Verification items for the finished model (mm, model axes). Face numbers are marked on the shaded views. A direction names the side the tool comes from. Round coordinates to 2 decimals unless told otherwise and drop trailing zeros. Loops run counter-clockwise (first coordinate to the right, second up) from the corner with the lowest first, then second, coordinate; pieces in that order, holes last. Notation, with made-up numbers: (29.5, 42) - (75.5, 42) arc R26 cw to (75.5, 74) - close; hole circle Ø6 at (61, 62.5). An arc over 180 degrees is marked (long way). Use CSV: the item, a comma, the result in double quotes.
Autodesk Inventor part; units mm, degrees
ref_plane "Work Plane1" through (1.525, 0, 0) normal (0, 0, 1) x (1, 0, 0)
ref_plane "YZ Plane" through (0, 0, 0) normal (1, 0, 0) x (0, 1, 0)
ref_plane "XZ Plane" through (0, 0, 0) normal (0, 1, 0) x (-1, 0, 0)
sketch "Sketch1" plane through (0, 0, 0) normal (0, 0, 1) x (1, 0, 0)
  line L0 (0, 14.1) -> (0, 10)
  line L1 (49, 10) -> (95, 10)
  line L2 (95, 10) -> (95, 0)
  line L3 (95, 0) -> (-0.8001, 0)
  line L4 (-19.9601, 0) -> (114.16, 0)
  line L5 (-0.8001, 0) -> (-0.8001, 14.1)
  line L6 (-0.8001, 14.1) -> (0, 14.1)
  line L7 (49, 10) -> (47.4663, 10)
  line L8 (47.4663, 10) -> (0, 10)
  line L9 (0, -2.82) -> (0, 16.92)
  dimension "d0" = 95
  dimension "d1" = 46
  dimension "d2" = 20
  dimension "d9" = 0.8001
  dimension "d10" = 28.2
  dimension "d13" = 1.5337
  dimension "d14" = 20
revolve "Body" add sketch "Sketch1" angle 360 about axis through (95, 0, 0) along (-1, 0, 0)
sketch "Sketch2" plane through (-0.8001, 0, 0) normal (-1, 0, 0) x (0, 0, 1)
  line L0 (0, 17.3205) -> (15, 8.6603)
  line L1 (15, 8.6603) -> (15, -8.6603)
  line L2 (15, -8.6603) -> (0, -17.3205)
  line L3 (0, -17.3205) -> (-15, -8.6603)
  line L4 (-15, -8.6603) -> (-15, 8.6603)
  line L5 (-15, 8.6603) -> (0, 17.3205)
  point P0 (0, 0)
  point P1 (0, 0)
  dimension "d11" = 30
extrude "Head" add sketch "Sketch2" along normal blind 11.7
sketch "Sketch4" plane through (0, 0, 0) normal (0, 0, 1) x (1, 0, 0)
  line L0 (-12.5001, 15) -> (-12.5001, 17.3205)
  line L1 (-12.5001, 17.3205) -> (-11.1604, 17.3205)
  line L2 (-11.1604, 17.3205) -> (-12.5001, 15)
  line L3 (-14.8401, 0) -> (1.5399, 0)
  line L4 (-0.8001, 17.3205) -> (-12.5001, 17.3205)
  line L5 (-12.5001, 8.6603) -> (-12.5001, 17.3205)
  dimension "d5" = 30
  dimension "d19" = 30
revolve "Chamfer1" cut sketch "Sketch4" angle 360 about axis through (-10, 0, 0) along (1, 0, 0)
thread "Thread"
chamfer "Chamfer2" distance 1.5336 distance2 1.5337 1 edges at (95, -10, 0) measured on face at (95, -2.495, 2.2104)
ref_plane "Work Plane1" through (1.525, 0, 0) normal (0, 0, 1) x (1, 0, 0)
equation "\"d0\" = NLG"
equation "\"d1\" = GEL"
equation "\"d2\" = GD"
equation "\"d10\" = SD2"
equation "\"d14\" = BDM"
equation "\"d11\" = SW"
equation "\"d3\" = KOH - SD"
equation "\"d5\" = ANG1"
equation "\"d19\" = SW0"
equation "\"d15\" = GEL"
equation "\"d6\" = -0.5 * SPD + 0.5 * GD"
equation "\"NLG\" = 95"
equation "\"GD\" = NND"
equation "\"BDM\" = NND"
equation "\"KOH\" = 12.5"
equation "\"GEL\" = 46"
equation "\"SW\" = 30"
equation "\"SW0\" = SW"
equation "\"SPD\" = NND - 1.2269 * PTC"
equation "\"SD2\" = 28.2"
equation "\"SD\" = 0.8"
equation "\"ANG1\" = 30deg"
equation "\"GAL\" = 0.61345 * PTC"
equation "\"GUL\" = 0.61345 * PTC"
equation "\"RR\" = 0.8"
equation "\"WFT\" = SD"
equation "\"GD1\" = THREADDIA - 1.2269 * PTC"
equation "\"SDH\" = 28.2"
equation "\"TOA\" = 30deg"
equation "\"FAWI\" = 45deg"
equation "\"PTC\" = 2.5"
equation "\"E0\" = 1.155 * SW"
properties part number "Bolt M20x95-8.8-A PN-85/M-82101" material "Steel, Mild"
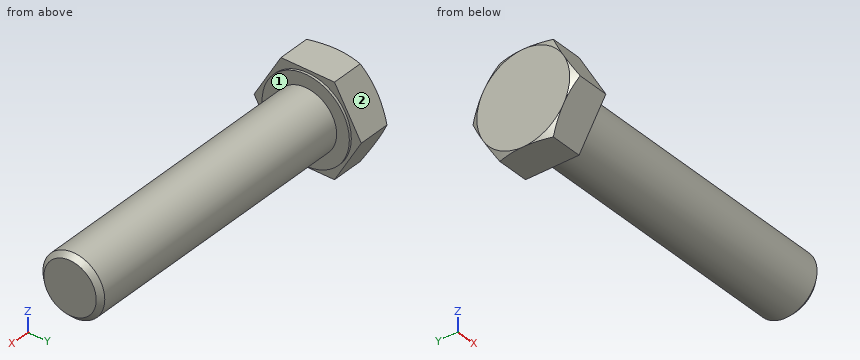
1) Access from +Z, -Z, +X, -X, +Y, -Y to the whole of each face (thin tool, end or side, straight path). Record for the marked faces 1 and 2.
Returned:
face 1,"+X"
face 2,"+Z, +X, -X, +Y"
2) Cross-section at A-A, the plane x = 36.5. Record the cut outline in (y, z).
Returned:
outline,"circle Ø20 at (0, 0)"
3) Gauge pin test, flat ends, axial feed: pin 1 Ø8 at (x, z) = (36.5, -10) entering from +Y; pin 2 Ø10 at (x, y) = (0, -13.5) entering from -Z; pin 3 Ø12 at (x, z) = (40.5, -5) entering from +Y; pin 4 Ø4 at (x, z) = (68.5, 11) entering from -Y. Record the tip position at first contact, or that the pin passes through.
Returned:
pin 1,"stops at y = 8"
pin 2,"stops at z = -15"
pin 3,"stops at y = 10"
pin 4,"stops at y = -4.36"
4) Thickness scan on probe 1 along X at (y, z) = (0, -11); probe 2 along X at (y, z) = (-14, 5); probe 3 along Y at (x, z) = (63, -0.5). Record the ranges inside material, lowest first. Write a range as [from, to].
Returned:
probe 1,"x = [-12.5, 0]"
probe 2,"x = [-12.5, -0.8]"
probe 3,"y = [-9.99, 9.99]"
